```python
from build123d import *

# Parameters (mm, degrees)
SKETCH1_R           = 75.565
SKETCH1_W           = 104.775
SKETCH1_H           = 10
BOSS_EXTRUDE1_DEPTH = 12.7
CUT_EXTRUDE1_DEPTH  = 12.7


with BuildPart() as part:
    # Sketch1 → Boss-Extrude1 (new body)
    with BuildSketch(Plane.XY):
        Circle(SKETCH1_R)
        with BuildLine():
            Line((-52.3875, 14.055637656), (52.3875, 14.055637656))
            ThreePointArc((52.3875, 14.055637656), (0, 54.240308869), (-52.3875, 14.055637656))
        make_face(mode=Mode.SUBTRACT)
        with Locations((0, -6.35)):
            Rectangle(SKETCH1_W, SKETCH1_H, mode=Mode.SUBTRACT)
        with BuildLine():
            Line((-52.3875, -23.154456235), (52.3875, -23.154456235))
            ThreePointArc((52.3875, -23.154456235), (0, -57.276338917), (-52.3875, -23.154456235))
        make_face(mode=Mode.SUBTRACT)
    extrude(amount=BOSS_EXTRUDE1_DEPTH)

    # Sketch3 → Cut-Extrude1 (cut)
    with BuildSketch(Plane.XY.offset(12.7)):
        Polygon((47.146344636, 60.616728817), (60.616728817, 47.146344636), (51.636472696, 38.166088515), (38.166088515, 51.636472696), align=None)
        Polygon((-52.534498308, -39.064114127), (-39.064114127, -52.534498308), (-48.044370248, -61.514754429), (-61.514754429, -48.044370248), align=None)
    extrude(amount=-CUT_EXTRUDE1_DEPTH, mode=Mode.SUBTRACT)


solid = part.part
```
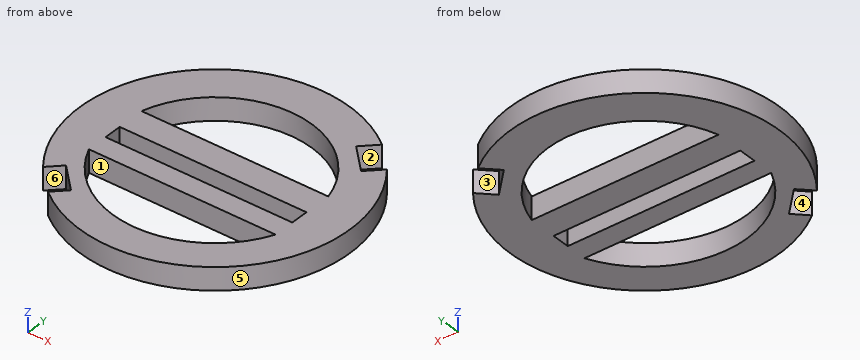
The model under review builds one solid part; all positions refer to its coordinate system, in mm. Face numbers are marked on the shaded views. A direction names the side the tool comes from. Give positions to 0.01 mm unless a question says otherwise; leave off trailing zeros. Write each loop counter-clockwise with the first axis right and the second up, starting at its lowest first coordinate (ties: lowest second). Pieces come first, ordered by that corner, then holes. Notation, with made-up numbers: M -21,83.5 L 4,83.5 A24 cw 4,96.5 Z; hole C 89,75 d2. An arc over 180 degrees is marked long. Write item = value, one per line. Start each with the question number.
Q1. We need section B-B (z = 5.75). Give the number of separate pieces and of enclosed holes in the cut face, plus the area to 3 significant figures.
Q2. Mouldability with a two-part tool opening along Y and no side actions: class the marked faces 4, 5 and 6 as released by +Y, released by -Y, zero draft, split by the parting line, or undercut.
Q3. We need section C-C (y = 33). State the section outline as (x, z) points, plus the area to 3 significant figures.
Q4. We need section D-D (x = 17.5). State the section outline as (y, z) points.
Q5. We need section A-A (y = -43). State the section outline as (x, z) points.
Q6. Machinability: for the marked faces 1, 2 and 3, which of the approach directions +Z, -Z, +X, -X, +Y, -Y give a long, thin tool a straight path to every point of the face, cutting with its end or side? Answer none if there is none.
Q7. Clearance check with flat-ended pins moving along their axes: pin 1 (4 mm diameter, centred on x = 8.5, z = 5, fed in from +Y); pin 2 (1 mm diameter, centred on y = -2.5, z = 8, fed in from +X); pin 3 (4 mm diameter, centred on x = -18, z = 9, fed in from -Y). State where each tip first meets the part, or that it passes through.
Q8. For line 1 (Y direction, x = -16.5, z = 1); line 2 (Y direction, x = 10, z = 3.25); line 3 (Y direction, x = -42.5, z = 7.25), list the stretches that pass through material, from the lowest coordinate up.
Result set:
q1.separate_pieces = 1
q1.enclosed_holes = 3
q1.area = 10,800 mm2
q2.face_4 = undercut
q2.face_5 = split by the parting line
q2.face_6 = released by -Y
q3.outline = M -67.98,0 L -43.05,0 L -43.05,12.7 L -67.98,12.7 Z; M 43.05,0 L 67.98,0 L 67.98,12.7 L 43.05,12.7 Z
q3.area = 633 mm2
q4.outline = M -73.51,0 L -54.54,0 L -54.54,12.7 L -73.51,12.7 Z; M -23.15,0 L -11.35,0 L -11.35,12.7 L -23.15,12.7 Z; M -1.35,0 L 14.06,0 L 14.06,12.7 L -1.35,12.7 Z; M 51.34,0 L 73.51,0 L 73.51,12.7 L 51.34,12.7 Z
q5.outline = M -62.14,0 L -56.47,0 L -56.47,12.7 L -62.14,12.7 Z; M -48.6,0 L -37.84,0 L -37.84,12.7 L -48.6,12.7 Z; M 37.84,0 L 62.14,0 L 62.14,12.7 L 37.84,12.7 Z
q6.face_1 = +Z, -Z
q6.face_2 = +Z, -Z, +X
q6.face_3 = +Z, -Z, +Y
q7.pin_1 = 75.28
q7.pin_2 = 75.54
q7.pin_3 = -73.85
q8.line_1 = -73.74 to -54.85, -23.15 to -11.35, -1.35 to 14.06, 51.67 to 73.74
q8.line_2 = -74.9 to -56.4, -23.15 to -11.35, -1.35 to 14.06, 53.31 to 74.9
q8.line_3 = -62.48 to -55.97, -49.1 to -38.4, -23.15 to -11.35, -1.35 to 14.06, 33.7 to 62.48
